from build123d import *

# Parameters (mm, degrees)
F0_W     = 1500
F0_H     = 20
F1_DEPTH = 15
F3_DEPTH = 25
F4_W     = 1500
F4_H     = 20
F5_DEPTH = 4
F6_R     = 4
F7_DEPTH = 20.001


with BuildPart() as f1:
    # F0 (on Front) → F1 (new body)
    with BuildSketch(Plane.XZ):
        Rectangle(F0_W, F0_H)
    extrude(amount=F1_DEPTH)

    # F2 (on face) → F3 (cut)
    with BuildSketch(Plane(origin=(0, 0, 0), x_dir=(-1, 0, 0), z_dir=(0, 1, 0))):
        Polygon((-736, 4), (-750, -10), (750, -10), (736, 4), align=None)
    extrude(amount=-F3_DEPTH, mode=Mode.SUBTRACT)

    # F4 (on face) → F5 (join)
    with BuildSketch(Plane(origin=(0, 0, 0), x_dir=(-1, 0, 0), z_dir=(0, 1, 0))):
        Rectangle(F4_W, F4_H)
    extrude(amount=F5_DEPTH)

    # F6 (on face) → F7 (cut, through all)
    with BuildSketch(Plane.XY.offset(10)):
        with Locations((-742, -5.5)):
            Circle(F6_R)
        with Locations((742, -5.5)):
            Circle(F6_R)
    extrude(amount=-F7_DEPTH, mode=Mode.SUBTRACT)


solid = f1.part
For this review, take the finished solid that the model builds, in its own axes (mm). Round coordinates to 2 decimals unless told otherwise and drop trailing zeros. Loops run counter-clockwise (first coordinate to the right, second up) from the corner with the lowest first, then second, coordinate; pieces in that order, holes last. Notation, with made-up numbers: (58, -12.5) - (98, -12.5) arc R25 cw to (98, -0.5) - close; hole circle Ø7 at (-24.75, 21.25). An arc over 180 degrees is marked (long way). Put each result on its own line as item: value. Start each with the question number.
1. Insertion check: P1, Ø6, axis at x = -23.5, z = -2.5, coming from the -Y side; P2, Ø2, axis at x = 22.5, y = -5.5, coming from the -Z side. Each pin has a flat end and moves straight along its axis. Give the tip position at first contact, or say it passes through.
2. Consider section C-C on z = -1.75. State the section outline as (x, y) points.
3. Consider section A-A on y = -5.5. State the section outline as (x, z) points.
4. Consider section B-B on x = 105.5. State the section outline as (y, z) points, plus the area to 3 significant figures.
5. For probe 1 along X at (y, z) = (-5.5, 4.5); probe 2 along Y at (x, z) = (742, 6); probe 3 along X at (y, z) = (-5.5, 1.75), list the stretches that pass through material, from the lowest coordinate up. Write a range as [from, to].
Result sheet:
1. P1: y = 0
1. P2: z = 4
2. outline: (-750, -15) - (-741.75, -15) - (-741.75, -9.49) arc R4 cw (long way) to (-741.75, -1.51) - (-741.75, 0) - (741.75, 0) - (741.75, -1.51) arc R4 cw (long way) to (741.75, -9.49) - (741.75, -15) - (750, -15) - (750, 4) - (-750, 4) - close
3. outline: (-750, -10) - (-746, -6) - (-746, 10) - (-750, 10) - close; (-738, 2) - (-736, 4) - (736, 4) - (738, 2) - (738, 10) - (-738, 10) - close; (746, -6) - (750, -10) - (750, 10) - (746, 10) - close
4. outline: (-15, 4) - (0, 4) - (0, -10) - (4, -10) - (4, 10) - (-15, 10) - close
4. area: 170 mm^2
5. probe 1: [-750, -746], [-738, 738], [746, 750]
5. probe 2: [-15, -9.5], [-1.5, 4]
5. probe 3: [-750, -746], [746, 750]
